The model under review builds one solid part; all positions refer to its coordinate system, in mm. A direction names the side the tool comes from. Round coordinates to 2 decimals unless told otherwise and drop trailing zeros. Order: outer loops, then holes, each group sorted by start corner. A loop starts at its lowest first (then second) coordinate and runs counter-clockwise, first axis right, second up. Notation, with made-up numbers: (57.25, 84) -> (106.25, 84) arc R20 cw to (106.25, 117) -> close; hole circle Ø7 at (-11.75, 36.25). An arc over 180 degrees is marked (long way). Return JSON: item names as keys, results as strings. Group by question number.
from build123d import *

# Parameters (mm, degrees)
SKETCH1_W           = 180
SKETCH1_H           = 230
SKETCH1_W_2         = 150
SKETCH1_H_2         = 200
BOSS_EXTRUDE1_DEPTH = 100
SKETCH2_W           = 180
SKETCH2_H           = 230
BOSS_EXTRUDE2_DEPTH = 15
SKETCH3_W           = 15
SKETCH3_H           = 70
BOSS_EXTRUDE3_DEPTH = 15
SKETCH4_W           = 60.52486508
SKETCH4_H           = 10.102082312
CUT_EXTRUDE1_DEPTH  = 10
SKETCH5_W           = 17.690019853
SKETCH5_H           = 44.485196982
CUT_EXTRUDE2_DEPTH  = 20


with BuildPart() as part:
    # Sketch1 → Boss-Extrude1 (new body)
    with BuildSketch(Plane(origin=(0, 0, 0), x_dir=(1, 0, 0), z_dir=(0, 1, 0))):
        Rectangle(SKETCH1_W, SKETCH1_H)
        Rectangle(SKETCH1_W_2, SKETCH1_H_2, mode=Mode.SUBTRACT)
    extrude(amount=BOSS_EXTRUDE1_DEPTH)

    # Sketch2 → Boss-Extrude2 (add)
    with BuildSketch(Plane.XZ):
        Rectangle(SKETCH2_W, SKETCH2_H)
    extrude(amount=-BOSS_EXTRUDE2_DEPTH)

    # Sketch3 → Boss-Extrude3 (add)
    with BuildSketch(Plane(origin=(0, 100, 0), x_dir=(1, 0, 0), z_dir=(0, 1, 0))):
        with Locations((-82.5, 0.801504388)):
            Rectangle(SKETCH3_W, SKETCH3_H)
    extrude(amount=BOSS_EXTRUDE3_DEPTH)

    # Sketch4 → Cut-Extrude1 (cut)
    with BuildSketch(Plane(origin=(-75, 0, 0), x_dir=(0, 0, -1), z_dir=(1, 0, 0))):
        with Locations((1.039053478, 105.051041156)):
            Rectangle(SKETCH4_W, SKETCH4_H)
    extrude(amount=-CUT_EXTRUDE1_DEPTH, mode=Mode.SUBTRACT)

    # Sketch5 → Cut-Extrude2 (cut)
    with BuildSketch(Plane(origin=(90, 0, 0), x_dir=(0, 0, -1), z_dir=(1, 0, 0))):
        with Locations((-76.613394803, 50.215874178)):
            Rectangle(SKETCH5_W, SKETCH5_H)
    extrude(amount=-CUT_EXTRUDE2_DEPTH, mode=Mode.SUBTRACT)


solid = part.part
Item 1: Consider section C-C on x = 63. State the section outline as (y, z) points.
Item 2: Consider section A-A on z = 79. State the section outline as (x, y) points, plus the area to 3 significant figures.
Item 3: Consider section D-D on y = 44.5. State the section outline as (x, z) points, plus the area to 3 significant figures.
Item 4: Consider section B-B on y = 93. State the section outline as (x, z) points.
Item 5: Wall thickness on line 1 along X through (y, z) = (17, -2.5); line 2 along Z through (x, y) = (-28, 21.5); line 3 along Y through (x, z) = (-78, 3): over which ranges is each line inside the solid? List them lowest first.
Item 6: For faces 4 (the face through (83, 50, 85.458)), 5 (the face through (-1, 49, -115)), 6 (the face through (-90, 57, 2)), 7 (the face through (-75, 53, 1)), 8 (the face through (-83, 107, 34.198)), list the 3-axis set-ups (+Z, -Z, +X, -X, +Y, -Y) from which the entire face can be reached by the end or side of a thin tool; tool diameter is ignored.
Item 7: Insertion check: pin 1 Ø7.5 at (x, y) = (-82, 107) entering from -Z; pin 2 Ø11 at (y, z) = (106, -4) entering from +X; pin 3 Ø4.5 at (x, z) = (86, 72.5) entering from +Y. Each pin has a flat end and moves straight along its axis. Give the tip position at first contact, or say it passes through.
Item 8: The part is to be moulded in two halves that separate along Z. For faces 1 (the face through (-1, 49, 115)), 2 (the face through (-85, 105, -1)), 3 (the face through (80, 100, -9)), say which applies: +Z half, -Z half, draft (parallel to the pull), parting line (faces both ways), or undercut.
Values:
{
 "1": {"outline": "(0, -115) -> (100, -115) -> (100, -100) -> (15, -100) -> (15, 100) -> (100, 100) -> (100, 115) -> (0, 115) -> close"},
 "2": {"outline": "(-90, 0) -> (90, 0) -> (90, 27.97) -> (75, 27.97) -> (75, 15) -> (-75, 15) -> (-75, 100) -> (-90, 100) -> close; (75, 72.46) -> (90, 72.46) -> (90, 100) -> (75, 100) -> close", "area": "4,580 mm^2"},
 "3": {"outline": "(-90, -115) -> (90, -115) -> (90, 67.77) -> (75, 67.77) -> (75, -100) -> (-75, -100) -> (-75, 100) -> (75, 100) -> (75, 85.46) -> (90, 85.46) -> (90, 115) -> (-90, 115) -> close", "area": "11,100 mm^2"},
 "4": {"outline": "(-90, -115) -> (90, -115) -> (90, 115) -> (-90, 115) -> close; hole (-75, -100) -> (75, -100) -> (75, 100) -> (-75, 100) -> close"},
 "5": {"line 1": "-90 to -75, 75 to 90", "line 2": "-115 to -100, 100 to 115", "line 3": "0 to 100, 110.1 to 115"},
 "6": {"face 4": "+X", "face 5": "-Z, +X, -X, +Y, -Y", "face 6": "+Z, -Z, -X, +Y, -Y", "face 7": "+Y", "face 8": "+Z, +X, -X, +Y"},
 "7": {"pin 1": "z = -35.8", "pin 2": "x = -75", "pin 3": "y = 100"},
 "8": {"face 1": "+Z half", "face 2": "undercut", "face 3": "draft"}
}
